The listing builds one solid part. Answer for the finished solid, in the listing's coordinates (mm). Face numbers are marked on the shaded views. A direction names the side the tool comes from. Give positions to 0.01 mm unless a question says otherwise; leave off trailing zeros. Order: outer loops, then holes, each group sorted by start corner. A loop starts at its lowest first (then second) coordinate and runs counter-clockwise, first axis right, second up. Notation, with made-up numbers: (10.5, 29) -> (43.5, 29) arc R12 cw to (43.5, 47) -> close; hole circle Ø11 at (18, -14.5). An arc over 180 degrees is marked (long way). One line per question, with ' | ' between items. Start each with the question number.
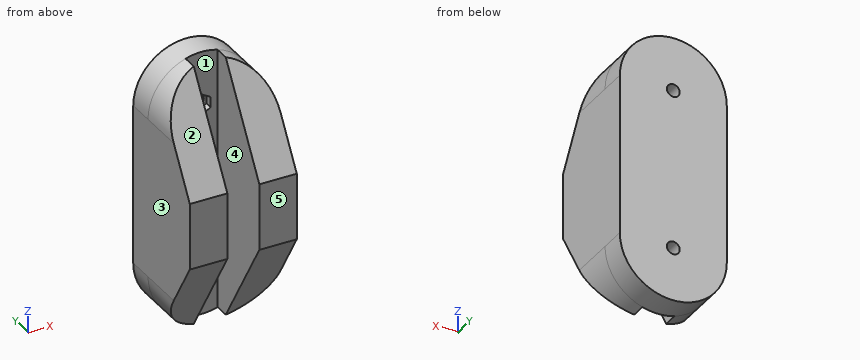
```python
from build123d import *

# Parameters (mm, degrees)
BOSS_EXTRUDE1_DEPTH      = 6.35
BOSS_EXTRUDE3_DEPTH      = 12.7
BOSS_EXTRUDE3_DEPTH_BACK = 12.7
CUT_EXTRUDE13_DEPTH      = 58.729461394
CUT_EXTRUDE13_DEPTH_BACK = 58.729461394
SKETCH11_W               = 7.59470995
SKETCH11_H               = 29.201393096
CUT_EXTRUDE19_DEPTH      = 56.356413171
CUT_EXTRUDE20_DEPTH      = 1.778
SKETCH17_R               = 1.524
CUT_EXTRUDE21_DEPTH      = 56.958411062


with BuildPart() as part:
    # Sketch1 → Boss-Extrude1 (new body)
    with BuildSketch(Plane(origin=(0, 0, 0), x_dir=(1, 0, 0), z_dir=(0, 1, 0))):
        with BuildLine():
            Line((12.7, 0), (12.7, -38.1))
            ThreePointArc((12.7, -38.1), (0, -50.8), (-12.7, -38.1))
            Line((-12.7, -38.1), (-12.7, 0))
            ThreePointArc((-12.7, 0), (0, 12.7), (12.7, 0))
        make_face()
    extrude(amount=-BOSS_EXTRUDE1_DEPTH)

    # Sketch2 → Boss-Extrude3 (add, two sides: drawn at the far end of the back side and taken through both)
    with BuildSketch(Plane(origin=(0, 0, 0), x_dir=(0, 0, -1), z_dir=(1, 0, 0)).offset(-BOSS_EXTRUDE3_DEPTH_BACK)):
        Polygon((-50.8, -6.35), (12.7, -6.35), (12.7, -9.525), (-11.11884122, -24.305569585), (-26.99384122, -24.305569585), (-50.8, -9.525), align=None)
    extrude(amount=BOSS_EXTRUDE3_DEPTH + BOSS_EXTRUDE3_DEPTH_BACK)

    # Sketch11 → Cut-Extrude13 (cut, two sides: drawn at the far end of the back side and taken through both)
    with BuildSketch(Plane.XY.offset(-CUT_EXTRUDE13_DEPTH_BACK)):
        with Locations((0.012645025, -20.950696548)):
            Rectangle(SKETCH11_W, SKETCH11_H)
    extrude(amount=CUT_EXTRUDE13_DEPTH + CUT_EXTRUDE13_DEPTH_BACK, mode=Mode.SUBTRACT)

    # Sketch10 → Cut-Extrude19 (cut, through all)
    with BuildSketch(Plane(origin=(0, -6.35, 0), x_dir=(1, 0, 0), z_dir=(0, 1, 0))):
        with BuildLine():
            ThreePointArc((0, 12.7), (8.980256121, 8.980256121), (12.7, 0))
            Line((12.7, 0), (12.7, 12.7))
            Line((12.7, 12.7), (0, 12.7))
        make_face()
        with BuildLine():
            Line((12.7, -50.8), (12.7, -38.1))
            ThreePointArc((12.7, -38.1), (8.980256121, -47.080256121), (0, -50.8))
            Line((0, -50.8), (12.7, -50.8))
        make_face()
        with BuildLine():
            ThreePointArc((-12.7, 0), (-8.980256121, 8.980256121), (0, 12.7))
            Line((0, 12.7), (-12.7, 12.7))
            Line((-12.7, 12.7), (-12.7, 0))
        make_face()
        with BuildLine():
            Line((-12.7, -50.8), (0, -50.8))
            ThreePointArc((0, -50.8), (-8.980256121, -47.080256121), (-12.7, -38.1))
            Line((-12.7, -38.1), (-12.7, -50.8))
        make_face()
    extrude(amount=-CUT_EXTRUDE19_DEPTH, mode=Mode.SUBTRACT)

    # Sketch16 → Cut-Extrude20 (cut)
    with BuildSketch(Plane.XZ.offset(6.35)):
        Polygon((0, 2.504895139), (-2.169302824, 1.252447569), (-2.169302824, -1.252447569), (0, -2.504895139), (2.169302824, -1.252447569), (2.169302824, 1.252447569), align=None)
        Polygon((0, 40.493188159), (-2.169302824, 39.24074059), (-2.169302824, 36.735845451), (0, 35.483397882), (2.169302824, 36.735845451), (2.169302824, 39.24074059), align=None)
    extrude(amount=-CUT_EXTRUDE20_DEPTH, mode=Mode.SUBTRACT)

    # Sketch17 → Cut-Extrude21 (cut, through all)
    with BuildSketch(Plane.XZ.offset(4.572)):
        with Locations(Location((0, 38.1, 0), (0, 0, 270))):
            Circle(SKETCH17_R)
        with Locations(Location((0, 0, 0), (0, 0, 270))):
            Circle(SKETCH17_R)
    extrude(amount=-CUT_EXTRUDE21_DEPTH, mode=Mode.SUBTRACT)


solid = part.part
```
(1) The part is cut by section C-C on x = 8.25. Determine the outline of the cut face in (y, z).
(2) Consider line 1 (X direction, y = -18, z = 34); line 2 (X direction, y = -3.35, z = 0); line 3 (Y direction, x = 1.75, z = -9.5). Determine where each line is inside the solid, lowest interval first.
(3) Given P1, Ø5, axis at x = 0, z = 38.1, coming from the -Y side; P2, Ø1, axis at x = -8.5, y = -18.5, coming from the -Z side; P3, Ø5, axis at x = -1, y = -18.5, coming from the -Z side; P4, Ø2, axis at x = -1, z = -0.5, coming from the -Y side, each flat-ended and moving along its own axis, determine where each tip first touches the part or whether it passes through.
(4) The part is cut by section B-B on z = 19. Determine the outline of the cut face in (x, y).
(5) Determine the mould class of the marked faces 1, 2 and 3 for opening direction X: pulls with the +X half, pulls with the -X half, needs draft (parallel to the pull), parting line crosses it, or undercut.
(6) The part is cut by section A-A on y = -7. Determine the outline of the cut face in (x, z), plus the area to 3 significant figures.
(7) The part is cut by section D-D on y = -15.75. Determine the outline of the cut face in (x, z).
(8) For the marked faces 4 and 5, determine the directions among +Z, -Z, +X, -X, +Y, -Y from which every point of the face is accessible in a straight line to the end or side of a thin tool.
Result sheet:
1) outline: (-24.31, 11.12) -> (-11.41, -9.66) -> (0, -9.66) -> (0, 47.76) -> (-11.42, 47.76) -> (-24.31, 26.99) -> close
2) line 1: x = -12.7 to -3.78, 3.81 to 12.7 | line 2: x = -12.7 to -1.52, 1.52 to 12.7 | line 3: y = -6.35 to 0
3) P1: stops at y = -6.35 | P2: stops at z = 0.96 | P3: passes through | P4: stops at y = -4.57
4) outline: (-12.7, -24.31) -> (-3.78, -24.31) -> (-3.78, -6.35) -> (3.81, -6.35) -> (3.81, -24.31) -> (12.7, -24.31) -> (12.7, 0) -> (-12.7, 0) -> close
5) face 1: undercut | face 2: needs draft | face 3: pulls with the -X half
6) outline: (-12.7, 0) arc R12.7 ccw to (-3.78, -12.12) -> (-3.78, 50.22) arc R12.7 ccw to (-12.7, 38.1) -> close; (3.81, -12.12) arc R12.7 ccw to (12.7, 0) -> (12.7, 38.1) arc R12.7 ccw to (3.81, 50.22) -> close | area: 995 mm^2
7) outline: (-12.7, 0) arc R12.7 ccw to (-12.42, -2.67) -> (-3.78, -2.67) -> (-3.78, 40.77) -> (-12.42, 40.77) arc R12.7 ccw to (-12.7, 38.1) -> close; (3.81, -2.67) -> (12.42, -2.67) arc R12.7 ccw to (12.7, 0) -> (12.7, 38.1) arc R12.7 ccw to (12.42, 40.77) -> (3.81, 40.77) -> close
8) face 4: +Z, -Z, -Y | face 5: +Z, -Z, +X, -X, -Y
